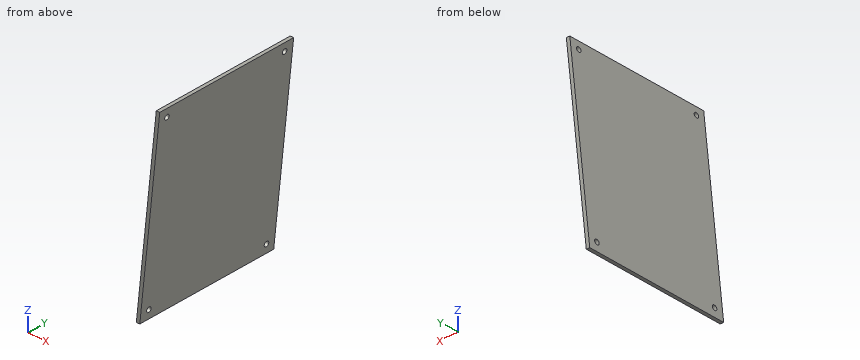
```python
from build123d import *

# Parameters (mm, degrees)
CYLINDER021_R               = 1.6
CYLINDER021_DEPTH           = 4
CYLINDER021_PLACEMENT_ANGLE = 96
CYLINDER022_R               = 1.6
CYLINDER022_DEPTH           = 4
CYLINDER022_PLACEMENT_ANGLE = 96
CYLINDER023_R               = 1.6
CYLINDER023_DEPTH           = 4
CYLINDER023_PLACEMENT_ANGLE = 96
CYLINDER020_R               = 1.6
CYLINDER020_DEPTH           = 4
CYLINDER020_PLACEMENT_ANGLE = 96
PAD_DEPTH                   = 94


with BuildPart() as loch2:
    # Cylinder021 → Cylinder021 (new body)
    with BuildSketch(Plane.XY):
        Circle(CYLINDER021_R)
    extrude(amount=CYLINDER021_DEPTH)


with BuildPart() as loch2_1:
    # Cylinder021 placement: moved
    add(loch2.part.moved(Location((10, 88.3, 116.5))).rotate(Axis((10, 88.3, 116.5), (0, 1, 0)), CYLINDER021_PLACEMENT_ANGLE))


with BuildPart() as loch3:
    # Cylinder022 → Cylinder022 (new body)
    with BuildSketch(Plane.XY):
        Circle(CYLINDER022_R)
    extrude(amount=CYLINDER022_DEPTH)


with BuildPart() as loch3_1:
    # Cylinder022 placement: moved
    add(loch3.part.moved(Location((-2.3, 88.3, 5.9))).rotate(Axis((-2.3, 88.3, 5.9), (0, 1, 0)), CYLINDER022_PLACEMENT_ANGLE))


with BuildPart() as loch4:
    # Cylinder023 → Cylinder023 (new body)
    with BuildSketch(Plane.XY):
        Circle(CYLINDER023_R)
    extrude(amount=CYLINDER023_DEPTH)


with BuildPart() as loch4_1:
    # Cylinder023 placement: moved
    add(loch4.part.moved(Location((10, 5.7, 116.5))).rotate(Axis((10, 5.7, 116.5), (0, 1, 0)), CYLINDER023_PLACEMENT_ANGLE))


with BuildPart() as l_cher:
    # Cylinder020 → Cylinder020 (new body)
    with BuildSketch(Plane.XY):
        Circle(CYLINDER020_R)
    extrude(amount=CYLINDER020_DEPTH)


with BuildPart() as l_cher_1:
    # Cylinder020 placement: moved
    add(l_cher.part.moved(Location((-2.3, 5.7, 5.9))).rotate(Axis((-2.3, 5.7, 5.9), (0, 1, 0)), CYLINDER020_PLACEMENT_ANGLE))

    # Fusion013: union Loch2, Loch3, Loch4
    add(loch2_1.part)
    add(loch3_1.part)
    add(loch4_1.part)


with BuildPart() as obj1:
    # Sketch003 → Pad (new body)
    with BuildSketch(Plane.XZ):
        Polygon((0, 0), (12.786083, 121.651457), (10.576083, 121.651457), (-2.21, 0), align=None)
    extrude(amount=-PAD_DEPTH)

    add(l_cher_1.part, mode=Mode.SUBTRACT)


solid = obj1.part
```
For this review, take the finished solid that the model builds, in its own axes (mm). Coordinates: 2 decimals unless noted, no trailing zeros. Order: outer loops, then holes, each group sorted by start corner. A loop starts at its lowest first (then second) coordinate and runs counter-clockwise, first axis right, second up. Notation, with made-up numbers: (43, 39) -> (60, 39) arc R34 cw to (60, 75) -> close; hole circle Ø3 at (-24, 6.25). An arc over 180 degrees is marked (long way). Use CSV: the item, a comma, the result in double quotes. Start each with the question number.
Item 1: Wall thickness on probe 1 along X at (y, z) = (41.5, 90.5); probe 2 along X at (y, z) = (17, 79.5): over which ranges is each line inside the solid? List them lowest first.
Item 2: We need section B-B, the plane z = 36. Give the boundary of the cut face in (x, y), then the cut area to 3 significant figures.
Item 3: We need section A-A, the plane y = 28.5. Give the boundary of the cut face in (x, z).
Item 4: Insertion check: pin 1 (12 mm diameter, centred on y = 37, z = 109, fed in from +X); pin 2 (8 mm diameter, centred on y = 24.5, z = 101, fed in from -X); pin 3 (5 mm diameter, centred on y = 76, z = 71.5, fed in from -X). Each pin has a flat end and moves straight along its axis. Give the tip position at first contact, or say it passes through.
Derived:
1,probe 1,"x = 7.3 to 9.51"
1,probe 2,"x = 6.15 to 8.36"
2,outline,"(1.57, 0) -> (3.78, 0) -> (3.78, 94) -> (1.57, 94) -> close"
2,area,"208 mm^2"
3,outline,"(-2.21, 0) -> (0, 0) -> (12.79, 121.65) -> (10.58, 121.65) -> close"
4,pin 1,"stops at x = 12.09"
4,pin 2,"stops at x = 7.99"
4,pin 3,"stops at x = 5.04"
